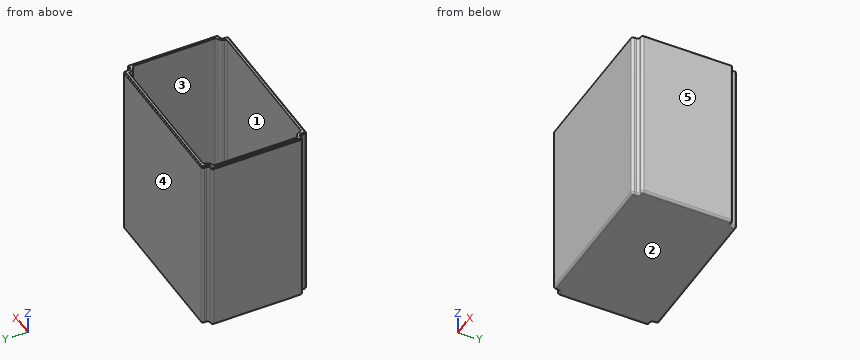
```python
from build123d import *

# Parameters (mm, degrees)
SKETCH_1_W      = 72
SKETCH_1_H      = 40.7
SKETCH_1_W_2    = 67
SKETCH_1_H_2    = 46.7
EXTRUDE_2_DEPTH = 80.6
FILLET_3_R      = 1
SHELL_START     = 1.5
SHELL_2_DEPTH   = 79.1
FILLET_4_R      = 1
FILLET_5_R      = 1
CHAMFER_1_SIZE  = 0.5
FILLET_6_R      = 1


# Read off the part's stored shape, not the designer's step: 抽壳2
with BuildPart() as part:
    # 草图1 → 凸台-拉伸2 (new body)
    with BuildSketch(Plane.XY):
        Rectangle(SKETCH_1_W, SKETCH_1_H)
        Rectangle(SKETCH_1_W_2, SKETCH_1_H_2)
    extrude(amount=EXTRUDE_2_DEPTH)

    # 圆角3
    fillet_3_edges = [part.edges().sort_by_distance(p)[0] for p in [
        (33.5, -20.35, 40.3),
        (-33.5, -20.35, 40.3),
        (-33.5, -23.35, 40.3),
        (33.5, -23.35, 40.3),
        (-36, -20.35, 40.3),
        (36, -20.35, 40.3),
        (36, 20.35, 40.3),
        (-36, 20.35, 40.3),
        (33.5, 20.35, 40.3),
        (-33.5, 20.35, 40.3),
        (-33.5, 23.35, 40.3),
        (33.5, 23.35, 40.3),
    ]]
    fillet(fillet_3_edges, radius=FILLET_3_R)

    # 抽壳2 outline → 抽壳2 (cut)
    with BuildSketch(Plane.XY.offset(SHELL_START)):
        with BuildLine():
            ThreePointArc((34.5, 18.85), (32.732233047, 19.582233047), (32, 21.35))
            Line((32, 21.35), (32, 21.85))
            Line((32, 21.85), (-32, 21.85))
            Line((-32, 21.85), (-32, 21.35))
            ThreePointArc((-32, 21.35), (-32.732233047, 19.582233047), (-34.5, 18.85))
            Line((-34.5, 18.85), (-34.5, -18.85))
            ThreePointArc((-34.5, -18.85), (-32.732233047, -19.582233047), (-32, -21.35))
            Line((-32, -21.35), (-32, -21.85))
            Line((-32, -21.85), (32, -21.85))
            Line((32, -21.85), (32, -21.35))
            ThreePointArc((32, -21.35), (32.732233047, -19.582233047), (34.5, -18.85))
            Line((34.5, -18.85), (34.5, 18.85))
        make_face()
    extrude(amount=SHELL_2_DEPTH, mode=Mode.SUBTRACT)

    # 圆角4
    fillet_4_edges = [part.edges().sort_by_distance(p)[0] for p in [
        (33.5, 21.85, 0),
        (34.75, 20.35, 0),
        (36, 0, 0),
        (34.75, -20.35, 0),
        (33.5, -21.85, 0),
        (0, -23.35, 0),
        (-33.5, -21.85, 0),
        (-34.75, -20.35, 0),
        (-36, 0, 0),
        (-34.75, 20.35, 0),
        (-33.5, 21.85, 0),
        (0, 23.35, 0),
        (35.707106781, -20.057106781, 0),
        (33.207106781, 23.057106781, 0),
        (-33.207106781, 23.057106781, 0),
        (-35.707106781, 20.057106781, 0),
        (-35.707106781, -20.057106781, 0),
        (-33.207106781, -23.057106781, 0),
        (33.207106781, -23.057106781, 0),
        (35.707106781, 20.057106781, 0),
        (33.792893219, 20.642893219, 0),
        (33.792893219, -20.642893219, 0),
        (-33.792893219, -20.642893219, 0),
        (-33.792893219, 20.642893219, 0),
    ]]
    fillet(fillet_4_edges, radius=FILLET_4_R)

    # 圆角5
    fillet_5_edges = [part.edges().sort_by_distance(p)[0] for p in [
        (34.5, 18.85, 41.05),
        (32, 21.85, 41.05),
        (32, 21.35, 41.05),
        (32, -21.85, 41.05),
        (32, -21.35, 41.05),
        (-32, 21.85, 41.05),
        (-32, 21.35, 41.05),
        (-32, -21.35, 41.05),
        (-32, -21.85, 41.05),
        (-34.5, 18.85, 41.05),
        (34.5, -18.85, 41.05),
        (-34.5, -18.85, 41.05),
    ]]
    fillet(fillet_5_edges, radius=FILLET_5_R)

    # 倒角1
    chamfer_1_edges = [part.edges().sort_by_distance(p)[0] for p in [
        (33.5, 21.85, 80.6),
        (34.75, 20.35, 80.6),
        (36, 0, 80.6),
        (0, 23.35, 80.6),
        (-33.5, 21.85, 80.6),
        (-34.75, 20.35, 80.6),
        (-36, 0, 80.6),
        (-34.75, -20.35, 80.6),
        (-33.5, -21.85, 80.6),
        (0, -23.35, 80.6),
        (33.5, -21.85, 80.6),
        (34.75, -20.35, 80.6),
        (35.707106781, -20.057106781, 80.6),
        (33.207106781, 23.057106781, 80.6),
        (-33.207106781, 23.057106781, 80.6),
        (-35.707106781, 20.057106781, 80.6),
        (-35.707106781, -20.057106781, 80.6),
        (-33.207106781, -23.057106781, 80.6),
        (33.207106781, -23.057106781, 80.6),
        (35.707106781, 20.057106781, 80.6),
        (33.792893219, 20.642893219, 80.6),
        (33.792893219, -20.642893219, 80.6),
        (-33.792893219, -20.642893219, 80.6),
        (-33.792893219, 20.642893219, 80.6),
    ]]
    chamfer(chamfer_1_edges, length=CHAMFER_1_SIZE)

    # 圆角6
    fillet_6_edges = [part.edges().sort_by_distance(p)[0] for p in [
        (32.607678605, 19.716255915, 1.5),
        (34.5, 0, 1.5),
        (0, 21.85, 1.5),
        (-32.607678605, 19.716255915, 1.5),
        (-34.5, 0, 1.5),
        (-32.607678605, -19.716255915, 1.5),
        (0, -21.85, 1.5),
        (32.607678605, -19.716255915, 1.5),
        (-34.301783726, -18.593512338, 1.5),
        (34.301783726, -18.593512338, 1.5),
        (31.690552056, -21.605928946, 1.5),
        (-31.690552056, -21.605928946, 1.5),
        (-34.301783726, 18.593512338, 1.5),
        (-31.690552056, 21.605928946, 1.5),
        (31.690552056, 21.605928946, 1.5),
        (34.301783726, 18.593512338, 1.5),
    ]]
    fillet(fillet_6_edges, radius=FILLET_6_R - 0.0001)  # a hair under: the kernel refuses the full size


solid = part.part
```
Read the model definition and answer for the solid it produces. Units are mm, in the model's axes. Face numbers are marked on the shaded views. A direction names the side the tool comes from. Coordinates: 2 decimals unless noted, no trailing zeros. Write each loop counter-clockwise with the first axis right and the second up, starting at its lowest first coordinate (ties: lowest second). Pieces come first, ordered by that corner, then holes. Notation, with made-up numbers: (59, 11.5) - (63, 11.5) arc R24 ccw to (63, 40.5) - close; hole circle Ø10 at (-8, 2.5). An arc over 180 degrees is marked (long way). Answer as a JSON object with one key per item and string values. Group by question number.
1. A cutting plane is placed at B-B (x = -5). Determine the outline of the cut face in (y, z).
2. Consider L1, parallel to Y at x = 28, z = 63.5; L2, parallel to X at y = 12, z = 7.5; L3, parallel to Z at x = -23, y = -12.5. Determine where each line is inside the solid, lowest interval first. Write a range as [from, to].
3. The mould has two halves that part along X. Classify the marked faces 3, 4 and 5: +X half, -X half, draft (parallel to the pull), parting line (faces both ways), or undercut.
4. Which of the six approach directions +Z, -Z, +X, -X, +Y, -Y give full straight-line access (tool end or side, diameter ignored) to the marked faces 1 and 2?
5. A cutting plane is placed at A-A (y = 12). Determine the outline of the cut face in (x, z).
6. Each of these flat-tipped pins is pushed along its axis until it touches: P1, Ø4, axis at x = -10, y = 2.5, coming from the +Z side; P2, Ø6, axis at x = -1.5, y = 13.5, coming from the -Z side; P3, Ø0.6, axis at x = -35, z = 23.5, coming from the -Y side; P4, Ø0.6, axis at x = -34.5, z = 39, coming from the +Y side. Where does it stop, or does it pass through?
Worked out:
{
 "1": {"outline": "(-23.35, 1) arc R1 ccw to (-22.35, 0) - (22.35, 0) arc R1 ccw to (23.35, 1) - (23.35, 80.1) - (22.85, 80.6) - (21.85, 80.6) - (21.85, 2.5) arc R1 cw to (20.85, 1.5) - (-20.85, 1.5) arc R1 cw to (-21.85, 2.5) - (-21.85, 80.6) - (-22.85, 80.6) - (-23.35, 80.1) - close"},
 "2": {"L1": "y = [-23.35, -21.85], [21.85, 23.35]", "L2": "x = [-36, -34.5], [34.5, 36]", "L3": "z = [0, 1.5]"},
 "3": {"face 3": "undercut", "face 4": "draft", "face 5": "+X half"},
 "4": {"face 1": "+Z", "face 2": "-Z, +X, -X, +Y, -Y"},
 "5": {"outline": "(-36, 1) arc R1 ccw to (-35, 0) - (35, 0) arc R1 ccw to (36, 1) - (36, 80.1) - (35.5, 80.6) - (34.5, 80.6) - (34.5, 2.5) arc R1 cw to (33.5, 1.5) - (-33.5, 1.5) arc R1 cw to (-34.5, 2.5) - (-34.5, 80.6) - (-35.5, 80.6) - (-36, 80.1) - close"},
 "6": {"P1": "stops at z = 1.5", "P2": "stops at z = 0", "P3": "stops at y = -20.35", "P4": "stops at y = 20.4"}
}
